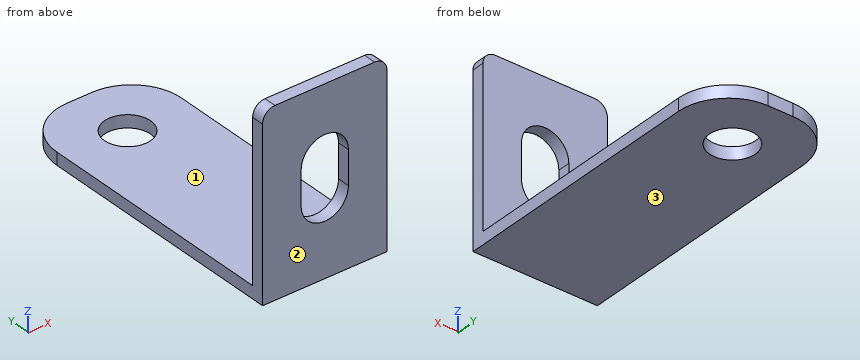
Autodesk Inventor part; units mm, degrees
ref_plane "YZ Plane" through (0, 0, 0) normal (1, 0, 0) x (0, 1, 0)
ref_plane "XZ Plane" through (0, 0, 0) normal (0, 1, 0) x (-1, 0, 0)
ref_plane "XY Plane" through (0, 0, 0) normal (0, 0, 1) x (1, 0, 0)
sketch "Sketch1" plane through (0, 0, 0) normal (0, 1, 0) x (-1, 0, 0)
  line L0 (5, 7.3) -> (-5, 7.3)
  line L1 (-5, 7.3) -> (-5, -7.3)
  line L2 (-5, -7.3) -> (5, -7.3)
  line L3 (5, -7.3) -> (5, 7.3)
  line L4 (5, 7.3) -> (-5, -7.3) construction
  line L5 (-5, 7.3) -> (5, -7.3) construction
  point P0 (0, 0)
  dimension "d0" = 10
  dimension "d1" = 14.6
extrude "Extrusion1" add sketch "Sketch1" along normal blind 1
sketch "Sketch2" plane through (5, 0, -7.3) normal (0, 0, -1) x (-1, 0, 0)
  line L0 (10, 0) -> (0, 0)
  line L1 (0, 0) -> (0, 24.7)
  line L2 (0, 24.7) -> (10, 24.7)
  line L3 (10, 24.7) -> (10, 0)
  point P0 (5, 0)
  dimension "d4" = 24.7
extrude "Extrusion2" add sketch "Sketch2" against normal blind 1
fillet "Fillet1" radius 4 2 edges at (5, 24.7, -6.8) (-5, 24.7, -6.8)
fillet "Fillet2" radius 1 2 edges at (-5, 0.5, 7.3) (5, 0.5, 7.3)
sketch "Sketch3" plane through (5, 0, -7.3) normal (0, 0, -1) x (-1, 0, 0)
  circle A0 centre (5, 19.85) radius 1.85
  line L0 (0, 0) -> (0, 20.7)
  line L1 (5, 21.7) -> (6.6441, 21.7) construction
  line L2 (4, 24.7) -> (6, 24.7) construction
  point P0 (5, 0)
  dimension "d9" = 3.7
  dimension "d10" = 5
  dimension "d11" = 3
extrude "Extrusion3" cut sketch "Sketch3" against normal blind 1
sketch "Sketch4" plane through (0, 0, 0) normal (0, -1, 0) x (1, 0, 0)
  arc A0 (1.9, 1.6) -> (-1.9, 1.6) centre (0, 1.6) ccw
  line L0 (-5, -7.3) -> (-5, 6.3)
  line L1 (-4, 7.3) -> (4, 7.3) construction
  line L2 (0, 3.5) -> (1.9, 3.5) construction
  arc A1 (-1.9, -1.1) -> (1.9, -1.1) centre (0, -1.1) ccw
  line L3 (0, -3) -> (1.9, -3) construction
  line L4 (1.9, 1.6) -> (1.9, -1.1)
  line L5 (-1.9, 1.6) -> (-1.9, -1.1)
  point P0 (0, 0)
  dimension "d14" = 3.8
  dimension "d15" = 5
  dimension "d17" = 3.8
  dimension "d18" = 3.8
  dimension "d19" = 6.5
  dimension "d20" = 5
extrude "Extrusion4" cut sketch "Sketch4" against normal blind 1
properties part number "Angle bracket long"
The listing builds one solid part. Answer for the finished solid, in the listing's coordinates (mm). Face numbers are marked on the shaded views. Round coordinates to 2 decimals unless told otherwise and drop trailing zeros. Write each loop counter-clockwise with the first axis right and the second up, starting at its lowest first coordinate (ties: lowest second). Pieces come first, ordered by that corner, then holes. Notation, with made-up numbers: M 76,-32 L 120,-32 A22 cw 120,-3 Z; hole C -40,16.5 d5. An arc over 180 degrees is marked long. Write each question's results on one line, items separated by ' | '. Start each with the question number.
Item 1: The mould has two halves that part along Z. Classify the marked faces 1, 2 and 3: +Z half, -Z half, draft (parallel to the pull), parting line (faces both ways), or undercut.
Item 2: Find section C-C on x = 0. Write down the section's boundary in (y, z), and give its area (3 significant figures).
Item 3: Find section B-B on y = 19.85. Write down the section's boundary in (x, z), and give its area (3 significant figures).
Item 4: Given pin 1 Ø5 at (y, z) = (13, -1.5) entering from +X; pin 2 Ø3 at (x, y) = (0, 16.5) entering from +Z; pin 3 Ø6 at (x, z) = (-3, 0) entering from +Y, each flat-ended and moving along its own axis, determine where each tip first touches the part or whether it passes through.
Item 5: Find section D-D on z = 4.25. Write down the section's boundary in (x, y).
Item 6: Find section A-A on z = -0.25. Write down the section's boundary in (x, y).
Item 7: Straight lines are drawn through the part: probe 1 along Y at (x, z) = (0, -6.8); probe 2 along Z at (x, y) = (0.25, 17.25); probe 3 along Y at (x, z) = (3.75, 6.75). For each, find the intervals that lie inside material, in ascending order.
Answer block:
1) face 1: +Z half | face 2: draft | face 3: -Z half
2) outline: M 0,-7.3 L 18,-7.3 L 18,-6.3 L 1,-6.3 L 1,-3 L 0,-3 Z; M 0,3.5 L 1,3.5 L 1,7.3 L 0,7.3 Z; M 21.7,-7.3 L 24.7,-7.3 L 24.7,-6.3 L 21.7,-6.3 Z | area: 28.1 mm²
3) outline: M -5,-7.3 L -1.85,-7.3 L -1.85,-6.3 L -5,-6.3 Z; M 1.85,-7.3 L 5,-7.3 L 5,-6.3 L 1.85,-6.3 Z | area: 6.30 mm²
4) pin 1: passes through | pin 2: stops at z = -6.3 | pin 3: stops at y = 1
5) outline: M -5,0 L 5,0 L 5,1 L -5,1 Z
6) outline: M -5,0 L -1.9,0 L -1.9,1 L -5,1 Z; M 1.9,0 L 5,0 L 5,1 L 1.9,1 Z
7) probe 1: y = 0 to 18, 21.7 to 24.7 | probe 2: z = -7.3 to -6.3 | probe 3: y = 0 to 1
